```python
from build123d import *

# Parameters (mm, degrees)
SKETCH1_W           = 120.5
SKETCH1_H           = 78
BOSS_EXTRUDE1_DEPTH = 1.5
CHAMFER1_SIZE       = 15
SKETCH2_W           = 81
SKETCH2_H           = 56
CUT_EXTRUDE1_DEPTH  = 2


with BuildPart() as part:
    # Sketch1 → Boss-Extrude1 (new body)
    with BuildSketch(Plane(origin=(0, 0, 0), x_dir=(1, 0, 0), z_dir=(0, 1, 0))):
        Rectangle(SKETCH1_W, SKETCH1_H)
    extrude(amount=BOSS_EXTRUDE1_DEPTH)

    # Chamfer1
    chamfer1_edges = [part.edges().sort_by_distance(p)[0] for p in [
        (60.25, 0.75, 39),
        (-60.25, 0.75, 39),
        (-60.25, 0.75, -39),
        (60.25, 0.75, -39),
    ]]
    chamfer(chamfer1_edges, length=CHAMFER1_SIZE)

    # Sketch2 → Cut-Extrude1 (cut)
    with BuildSketch(Plane(origin=(0, 1.5, 0), x_dir=(1, 0, 0), z_dir=(0, 1, 0))):
        Rectangle(SKETCH2_W, SKETCH2_H)
    extrude(amount=-CUT_EXTRUDE1_DEPTH, mode=Mode.SUBTRACT)


solid = part.part
```
For this review, take the finished solid that the model builds, in its own axes (mm). Round coordinates to 2 decimals unless told otherwise and drop trailing zeros. Loops run counter-clockwise (first coordinate to the right, second up) from the corner with the lowest first, then second, coordinate; pieces in that order, holes last.
(1) We need section B-B (z = -21.5). Give the boundary of the cut face in (x, y).
Returned:
outline: (-60.25, 0) - (-40.5, 0) - (-40.5, 1.5) - (-60.25, 1.5) - close; (40.5, 0) - (60.25, 0) - (60.25, 1.5) - (40.5, 1.5) - close
(2) Mouldability with a two-part tool opening along Y and no side actions: class faces 1 (the flat face through (52.855, 0.74, 31.395)), 2 (the flat face through (-41, 0, -1)), 3 (the flat face through (-41, 1.5, -1)) as released by +Y, released by -Y, zero draft, split by the parting line, or undercut.
Returned:
face 1: zero draft
face 2: released by -Y
face 3: released by +Y
(3) We need section A-A (x = 0.5). Give the boundary of the cut face in (y, z).
Returned:
outline: (0, -39) - (1.5, -39) - (1.5, -28) - (0, -28) - close; (0, 28) - (1.5, 28) - (1.5, 39) - (0, 39) - close
(4) Wall thickness on line 1 along X through (y, z) = (0.9, -9); line 2 along Z through (x, y) = (16.5, 0.5); line 3 along X through (y, z) = (1.3, 25): over which ranges is each line inside the solid? List them lowest first.
Returned:
line 1: x = -60.25 to -40.5, 40.5 to 60.25
line 2: z = -39 to -28, 28 to 39
line 3: x = -59.25 to -40.5, 40.5 to 59.25
(5) We need section C-C (y = 1.15). Give the boundary of the cut face in (x, z).
Returned:
outline: (-60.25, -24) - (-45.25, -39) - (45.25, -39) - (60.25, -24) - (60.25, 24) - (45.25, 39) - (-45.25, 39) - (-60.25, 24) - close; hole (-40.5, -28) - (40.5, -28) - (40.5, 28) - (-40.5, 28) - close
(6) We need section D-D (z = -31). Give the boundary of the cut face in (x, y), plus the area to 3 significant figures.
Returned:
outline: (-53.25, 0) - (53.25, 0) - (53.25, 1.5) - (-53.25, 1.5) - close
area: 160 mm2
